Input: part model. Units: mm. Frame: model coordinates. Face numbers are marked on the shaded views. Give positions to 0.01 mm unless a question says otherwise; leave off trailing zeros. Loops run counter-clockwise (first coordinate to the right, second up) from the corner with the lowest first, then second, coordinate; pieces in that order, holes last. Notation, with made-up numbers: (-32, 71) - (-22, 71) arc R22 cw to (-22, 93) - close; hole circle Ø5 at (23, -34.75). An arc over 180 degrees is marked (long way). Answer as a JSON object with one key per item and string values.
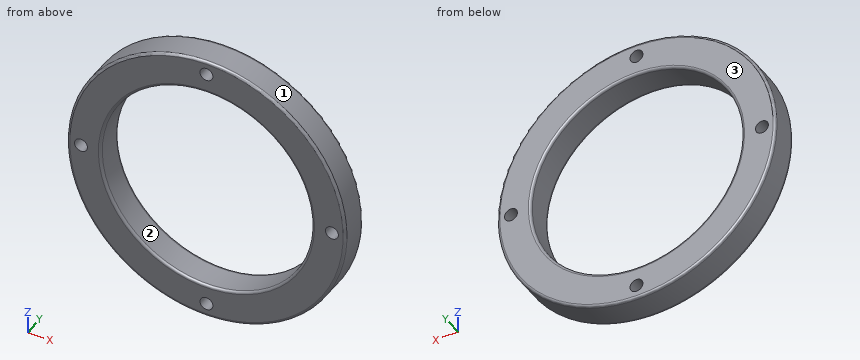
from build123d import *

# Parameters (mm, degrees)
SKETCH_3_R      = 56
SKETCH_3_R_2    = 42.5
SKETCH_3_R_3    = 2.6
EXTRUDE_1_DEPTH = 12
FILLET_1_R      = 1


with BuildPart() as part:
    # 草图3 → 凸台-拉伸1 (new body)
    with BuildSketch(Plane(origin=(0, 0, 0), x_dir=(1, 0, 0), z_dir=(0, 1, 0))):
        with Locations(Location((0, 0, 0), (0, 0, 270))):
            Circle(SKETCH_3_R)
        with Locations(Location((0, 0, 0), (0, 0, 270))):
            Circle(SKETCH_3_R_2, mode=Mode.SUBTRACT)
        with Locations(Location((50.5, 0, 0), (0, 0, 270))):
            Circle(SKETCH_3_R_3, mode=Mode.SUBTRACT)
        with Locations(Location((0, -50.5, 0), (0, 0, 270))):
            Circle(SKETCH_3_R_3, mode=Mode.SUBTRACT)
        with Locations(Location((-50.5, 0, 0), (0, 0, 270))):
            Circle(SKETCH_3_R_3, mode=Mode.SUBTRACT)
        with Locations(Location((0, 50.5, 0), (0, 0, 270))):
            Circle(SKETCH_3_R_3, mode=Mode.SUBTRACT)
    extrude(amount=EXTRUDE_1_DEPTH)

    # 圆角1
    fillet_1_edges = [part.edges().sort_by_distance(p)[0] for p in [
        (0, 0, -56),
        (0, 12, -56),
        (0, 0, -42.5),
        (0, 12, -42.5),
    ]]
    fillet(fillet_1_edges, radius=FILLET_1_R)


solid = part.part
Item 1: Material intervals for line 1 (X direction, y = 8.25, z = 0); line 2 (Z direction, x = 8.5, y = 3.75); line 3 (Z direction, x = -39, y = 1.25), sorted ascending. Write a range as [from, to].
Geometry check:
{"line 1": "x = [-56, -53.1], [-47.9, -42.5], [42.5, 47.9], [53.1, 56]", "line 2": "z = [-55.35, -41.64], [41.64, 55.35]", "line 3": "z = [-40.19, -16.89], [16.89, 40.19]"}
Item 2: Contact query for flat-ended pins moving along their axis: P1, Ø3, axis at x = 0, z = 50.5, coming from the -Y side; P2, Ø1, axis at x = -41.5, y = 9, coming from the +Z side; P3, Ø1, axis at y = 5, z = 29.5, coming from the -X side; P4, Ø1, axis at y = 5.5, z = 42.5, coming from the +X side. Output: stop coordinate, or through.
Geometry check:
{"P1": "passes through", "P2": "stops at z = 38.14", "P3": "stops at x = -47.91", "P4": "stops at x = 37.04"}
Item 3: Cut plane C-C (y = 8.5). Return loops of the section in (x, z), then the cut area to 3 significant figures.
Geometry check:
{"outline": "circle Ø112 at (0, 0); hole circle Ø5.2 at (-50.5, 0); hole circle Ø85 at (0, 0); hole circle Ø5.2 at (0, -50.5); hole circle Ø5.2 at (0, 50.5); hole circle Ø5.2 at (50.5, 0)", "area": "4,090 mm2"}
Item 4: Cut plane A-A (z = 0). Return loops of the section in (x, y).
Geometry check:
{"outline": "(-56, 1) arc R1 ccw to (-55, 0) - (-53.1, 0) - (-53.1, 12) - (-55, 12) arc R1 ccw to (-56, 11) - close; (-47.9, 0) - (-43.5, 0) arc R1 ccw to (-42.5, 1) - (-42.5, 11) arc R1 ccw to (-43.5, 12) - (-47.9, 12) - close; (42.5, 1) arc R1 ccw to (43.5, 0) - (47.9, 0) - (47.9, 12) - (43.5, 12) arc R1 ccw to (42.5, 11) - close; (53.1, 0) - (55, 0) arc R1 ccw to (56, 1) - (56, 11) arc R1 ccw to (55, 12) - (53.1, 12) - close"}
Item 5: Cut plane B-B (x = 0). Return loops of the section in (y, z), then the cut area to 3 significant figures.
Geometry check:
{"outline": "(0, -55) arc R1 ccw to (1, -56) - (11, -56) arc R1 ccw to (12, -55) - (12, -53.1) - (0, -53.1) - close; (0, -47.9) - (12, -47.9) - (12, -43.5) arc R1 ccw to (11, -42.5) - (1, -42.5) arc R1 ccw to (0, -43.5) - close; (0, 43.5) arc R1 ccw to (1, 42.5) - (11, 42.5) arc R1 ccw to (12, 43.5) - (12, 47.9) - (0, 47.9) - close; (0, 53.1) - (12, 53.1) - (12, 55) arc R1 ccw to (11, 56) - (1, 56) arc R1 ccw to (0, 55) - close", "area": "197 mm2"}
Item 6: Mould query, pull axis X, two halves, no side actions, for the marked faces 1, 2 and 3. Classes: released by +X, released by -X, zero draft, split by the parting line, or undercut.
Geometry check:
{"face 1": "split by the parting line", "face 2": "undercut", "face 3": "zero draft"}
